Source: CAD feature listing. Evaluate the final solid. Frame: model axes, mm. A direction names the side the tool comes from. Round coordinates to 2 decimals unless told otherwise and drop trailing zeros. Order: outer loops, then holes, each group sorted by start corner. A loop starts at its lowest first (then second) coordinate and runs counter-clockwise, first axis right, second up. Notation, with made-up numbers: (10.5, 31.5) - (56.5, 31.5) arc R18 cw to (56.5, 51.5) - close; hole circle Ø10 at (52.25, 79). An arc over 180 degrees is marked (long way). Use one line per item in the form item = value. Start each with the question number.
Q1. Cut plane C-C, the plane z = 16.5. Return the cut outline in (x, y), and give its area (3 significant figures).
Q2. Set-up query: faces 1 (the cylindrical face through (-50.56, 0.72, 17.49)), 2 (the flat face through (-32.5, 0, -17)). Return all of +Z, -Z, +X, -X, +Y, -Y with unobstructed straight access to the full face (end or side cutting, diameter ignored); none if empty.
Q3. Cut plane A-A, the plane x = 25. Return the cut outline in (y, z).
Q4. Cut plane D-D, the plane y = 44. Return the cut outline in (x, z).
Q5. Draft query along Z for faces 3 (the cylindrical face through (64.998, 0.784, -0.556)), 4 (the flat face through (37.5, 0, 18)), 5 (the flat face through (4, -1, -15)). Return one class per face: released by +Z, released by -Z, zero draft, split by the parting line, or undercut.
Q6. Ray query, line 1 (Z direction, x = 48.5, y = -29); line 2 (X direction, y = 16, z = 16.5); line 3 (Y direction, x = -36.5, z = -19). Return the intervals inside material, ascending. Write a range as [from, to].
Q7. Pin query (flat end, axial travel): pin 1 Ø5.5 at (x, z) = (35, 17) entering from -Y; pin 2 Ø2 at (x, y) = (-38, 40) entering from -Z; pin 3 Ø1.5 at (y, z) = (-6.5, 16.5) entering from +X. Return the tip coordinate at first contact, or that it passes through.
Q8. Cut plane B-B, the plane y = 31. Return the cut outline in (x, z), and give its area (3 significant figures).
from build123d import *

# Parameters (mm, degrees)
BOSS_EXTRUDE1_DEPTH = 56
BOSS_EXTRUDE2_DEPTH = 51.5
CUT_EXTRUDE1_REACH  = 105.161
SKETCH3_W           = 5
SKETCH3_H           = 65


with BuildPart() as part:
    # Sketch1 → Boss-Extrude1 (new, symmetric)
    with BuildSketch(Plane(origin=(0, 0, 0), x_dir=(1, 0, 0), z_dir=(0, 1, 0))):
        with BuildLine():
            Line((50.787426746, 35.561739054), (53.244882879, 37.282468363))
            ThreePointArc((53.244882879, 37.282468363), (65, 0), (53.244882879, -37.282468363))
            Line((53.244882879, -37.282468363), (50.787426746, -35.561739054))
            ThreePointArc((50.787426746, -35.561739054), (62, 0), (50.787426746, 35.561739054))
        make_face()
    extrude(amount=BOSS_EXTRUDE1_DEPTH, both=True)

    # Sketch2 → Boss-Extrude2 (add, symmetric)
    with BuildSketch(Plane(origin=(0, 0, 0), x_dir=(1, 0, 0), z_dir=(0, 1, 0))):
        with BuildLine():
            Line((-51.354162441, 15), (60.158124971, 15))
            ThreePointArc((60.158124971, 15), (59.474430807, 17.515481159), (58.685603004, 20))
            Line((58.685603004, 20), (-49.621064076, 20))
            ThreePointArc((-49.621064076, 20), (-50.549471733, 17.521441364), (-51.354162441, 15))
        make_face()
        with BuildLine():
            Line((-49.621064076, -20), (58.685603004, -20))
            ThreePointArc((58.685603004, -20), (59.474430807, -17.515481159), (60.158124971, -15))
            Line((60.158124971, -15), (-51.354162441, -15))
            ThreePointArc((-51.354162441, -15), (-50.549471733, -17.521441364), (-49.621064076, -20))
        make_face()
    extrude(amount=BOSS_EXTRUDE2_DEPTH, both=True)

    # Cut-Extrude1: up to this face of the body (flat: up to its plane)
    cut_extrude1_end = Plane(part.part.faces().sort_by_distance((4.532269464, 0, -20))[0])
    # Sketch3 → Cut-Extrude1 (cut, up to the picked face)
    with BuildSketch(Plane.XY.offset(20), mode=Mode.PRIVATE) as cut_extrude1_sk1:
        with Locations((-35, 0)):
            Rectangle(SKETCH3_W, SKETCH3_H)
    cut_extrude1_tool1 = split(extrude(cut_extrude1_sk1.sketch, amount=-CUT_EXTRUDE1_REACH, mode=Mode.PRIVATE), bisect_by=cut_extrude1_end, keep=Keep.BOTH, mode=Mode.PRIVATE)
    # Sketch3 → Cut-Extrude1 (cut, up to the picked face)
    with BuildSketch(Plane.XY.offset(20), mode=Mode.PRIVATE) as cut_extrude1_sk2:
        with Locations((35, 0)):
            Rectangle(SKETCH3_W, SKETCH3_H)
    cut_extrude1_tool2 = split(extrude(cut_extrude1_sk2.sketch, amount=-CUT_EXTRUDE1_REACH, mode=Mode.PRIVATE), bisect_by=cut_extrude1_end, keep=Keep.BOTH, mode=Mode.PRIVATE)
    add(cut_extrude1_tool1.solids().sort_by(Axis((-35, 0, 20), (0, 0, -1)))[0], mode=Mode.SUBTRACT)
    add(cut_extrude1_tool2.solids().sort_by(Axis((35, 0, 20), (0, 0, -1)))[0], mode=Mode.SUBTRACT)


solid = part.part
Completed:
q1.outline = (-50.89, -51.5) - (59.76, -51.5) - (59.76, -56) - (62.87, -56) - (62.87, 56) - (59.76, 56) - (59.76, 51.5) - (-50.89, 51.5) - close; hole (-37.5, -32.5) - (-32.5, -32.5) - (-32.5, 32.5) - (-37.5, 32.5) - close; hole (32.5, -32.5) - (37.5, -32.5) - (37.5, 32.5) - (32.5, 32.5) - close
q1.area = 11,100 mm2
q2.face_1 = +Z, -X, +Y, -Y
q2.face_2 = +Z, -Z
q3.outline = (-51.5, -20) - (51.5, -20) - (51.5, -15) - (-51.5, -15) - close; (-51.5, 15) - (51.5, 15) - (51.5, 20) - (-51.5, 20) - close
q4.outline = (-51.35, -15) arc R53.5 ccw to (-49.62, -20) - (58.69, -20) arc R62 cw to (50.79, -35.56) - (53.24, -37.28) arc R65 ccw to (53.24, 37.28) - (50.79, 35.56) arc R62 cw to (58.69, 20) - (-49.62, 20) arc R53.5 ccw to (-51.35, 15) - (60.16, 15) arc R62 cw to (60.16, -15) - close
q5.face_3 = split by the parting line
q5.face_4 = zero draft
q5.face_5 = undercut
q6.line_1 = [-20, -15], [15, 20]
q6.line_2 = [-50.89, -37.5], [-32.5, 32.5], [37.5, 62.87]
q6.line_3 = [-51.5, -32.5], [32.5, 51.5]
q7.pin_1 = -51.5
q7.pin_2 = -20
q7.pin_3 = 63.06
q8.outline = (-51.35, -15) arc R53.5 ccw to (-49.62, -20) - (-37.5, -20) - (-37.5, -15) - close; (-51.35, 15) - (-37.5, 15) - (-37.5, 20) - (-49.62, 20) arc R53.5 ccw to start; (-32.5, -20) - (32.5, -20) - (32.5, -15) - (-32.5, -15) - close; (-32.5, 15) - (32.5, 15) - (32.5, 20) - (-32.5, 20) - close; (37.5, -20) - (58.69, -20) arc R62 cw to (50.79, -35.56) - (53.24, -37.28) arc R65 ccw to (53.24, 37.28) - (50.79, 35.56) arc R62 cw to (58.69, 20) - (37.5, 20) - (37.5, 15) - (60.16, 15) arc R62 cw to (60.16, -15) - (37.5, -15) - close
q8.area = 1,230 mm2
